CAD build for the part. Positions are in the model's coordinates, mm. Face numbers are marked on the shaded views. A direction names the side the tool comes from. Give positions to 0.01 mm unless a question says otherwise; leave off trailing zeros. Loops run counter-clockwise (first coordinate to the right, second up) from the corner with the lowest first, then second, coordinate; pieces in that order, holes last.
Item 1: Which spindle directions (+Z, -Z, +X, -X, +Y, -Y) get a long thin tool onto all of the face, cutting with end or side? Do the marked faces 1 and 2. Say none if no direction does.
Item 2: Saw through at B-B on y = 168.5. Give the cut face in (x, z).
Item 3: Saw through at A-A on y = 43. Give the cut face in (x, z).
Item 4: Drop flat-ended pins along their axis: P1, Ø1.5, axis at y = 74.5, z = 22.5, coming from the +X side; P2, Ø22, axis at x = 27, y = 501, coming from the +Z side; P3, Ø0.9, axis at x = 2, y = 27, coming from the -Z side. Give the stop position or say it passes through.
Item 5: Saw through at C-C on x = 33.5. Give the cut face in (y, z), plus the area to 3 significant figures.
Item 6: Probe probe 1 along Z at (x, y) = (19, 164); probe 2 along X at (y, z) = (309, 4). List the from-to ranges inside material, lowest first.
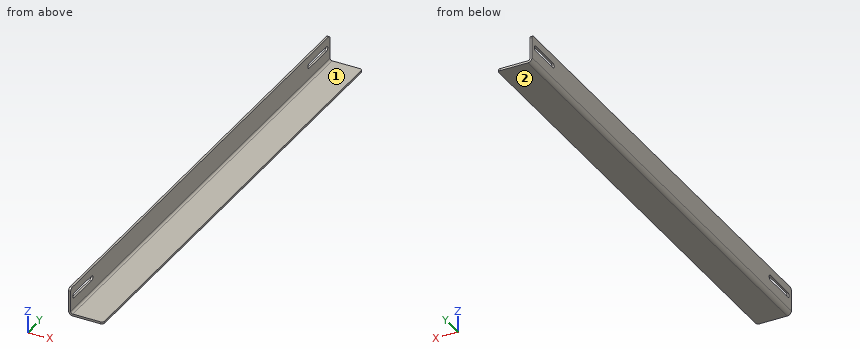
from build123d import *

# Parameters (mm, degrees)
F0_W      = 50
F0_H      = 40
F2_DEPTH  = 700
F1_W      = 47
F1_H      = 37
F3_DEPTH  = 700
F4_R      = 6
F5_R      = 3
F6_R      = 4
F7_R      = 4
F8_R      = 4
F9_R      = 4
F10_W     = 47
F10_H     = 7
F11_DEPTH = 3
F12_W     = 47
F12_H     = 7
F13_DEPTH = 3


with BuildPart() as f2:
    # F0 (on Front) → F2 (new body)
    with BuildSketch(Plane.XZ):
        with Locations((25, 20)):
            Rectangle(F0_W, F0_H)
    extrude(amount=-F2_DEPTH)

    # F1 (on face) → F3 (cut)
    with BuildSketch(Plane.XZ):
        with Locations((26.5, 21.5)):
            Rectangle(F1_W, F1_H)
    extrude(amount=-F3_DEPTH, mode=Mode.SUBTRACT)

    # F4
    f4_edges = [f2.edges().sort_by_distance(p)[0] for p in [
        (0, 350, 0),
    ]]
    fillet(f4_edges, radius=F4_R)

    # F5
    f5_edges = [f2.edges().sort_by_distance(p)[0] for p in [
        (3, 350, 3),
    ]]
    fillet(f5_edges, radius=F5_R)

    # F6
    f6_edges = [f2.edges().sort_by_distance(p)[0] for p in [
        (1.5, 0, 40),
    ]]
    fillet(f6_edges, radius=F6_R)

    # F7
    f7_edges = [f2.edges().sort_by_distance(p)[0] for p in [
        (1.5, 700, 40),
    ]]
    fillet(f7_edges, radius=F7_R)

    # F8
    f8_edges = [f2.edges().sort_by_distance(p)[0] for p in [
        (50, 0, 1.5),
    ]]
    fillet(f8_edges, radius=F8_R)

    # F9
    f9_edges = [f2.edges().sort_by_distance(p)[0] for p in [
        (50, 700, 1.5),
    ]]
    fillet(f9_edges, radius=F9_R)

    # F10 (on face) → F11 (cut)
    with BuildSketch(Plane(origin=(0, 0, 0), x_dir=(0, -1, 0), z_dir=(-1, 0, 0))):
        with Locations((-667, 25)):
            Rectangle(F10_W, F10_H)
        with BuildLine():
            Line((-690.5, 21.5), (-690.5, 28.5))
            ThreePointArc((-690.5, 28.5), (-694, 25), (-690.5, 21.5))
        make_face()
        with BuildLine():
            ThreePointArc((-643.5, 21.5), (-640, 25), (-643.5, 28.5))
            Line((-643.5, 28.5), (-643.5, 21.5))
        make_face()
    extrude(amount=-F11_DEPTH, mode=Mode.SUBTRACT)

    # F12 (on face) → F13 (cut)
    with BuildSketch(Plane(origin=(0, 0, 0), x_dir=(0, -1, 0), z_dir=(-1, 0, 0))):
        with Locations((-33, 25)):
            Rectangle(F12_W, F12_H)
        with BuildLine():
            Line((-56.5, 21.5), (-56.5, 28.5))
            ThreePointArc((-56.5, 28.5), (-60, 25), (-56.5, 21.5))
        make_face()
        with BuildLine():
            ThreePointArc((-9.5, 21.5), (-6, 25), (-9.5, 28.5))
            Line((-9.5, 28.5), (-9.5, 21.5))
        make_face()
    extrude(amount=-F13_DEPTH, mode=Mode.SUBTRACT)


solid = f2.part
Results below:
1. face 1: +Z, +X, +Y, -Y
1. face 2: -Z, +X, -X, +Y, -Y
2. outline: (0, 6) arc R6 ccw to (6, 0) - (50, 0) - (50, 3) - (6, 3) arc R3 cw to (3, 6) - (3, 40) - (0, 40) - close
3. outline: (0, 6) arc R6 ccw to (6, 0) - (50, 0) - (50, 3) - (6, 3) arc R3 cw to (3, 6) - (3, 21.5) - (0, 21.5) - close; (0, 28.5) - (3, 28.5) - (3, 40) - (0, 40) - close
4. P1: stops at x = 3
4. P2: stops at z = 3
4. P3: stops at z = 1.16
5. outline: (0, 0) - (700, 0) - (700, 3) - (0, 3) - close
5. area: 2,100 mm2
6. probe 1: z = 0 to 3
6. probe 2: x = 0.34 to 3.76
